Part model, mm, in its own coordinate system. Face numbers are marked on the shaded views. A direction names the side the tool comes from. Coordinates: 2 decimals unless noted, no trailing zeros. Write each loop counter-clockwise with the first axis right and the second up, starting at its lowest first coordinate (ties: lowest second). Pieces come first, ordered by that corner, then holes. Notation, with made-up numbers: M -33,-22 L 14,-22 A21 ccw 14,-13 Z; hole C 25,-22 d6. An arc over 180 degrees is marked long. Use a Markdown table: item, result. Add a question column.
Q1. Slice it at C-C on z = -27. Write the cut outline in (x, y), then the cut area to 3 significant figures.
Q2. Pin check, flat tips, straight feed: pin 1 Ø5 at (y, z) = (-17.5, -44.5) entering from -X; pin 2 Ø18.5 at (x, z) = (20, -32.5) entering from -Y. Stop position of each tip, or through.
Q3. Slice it at D-D on y = -11. Write the cut outline in (x, z), then the cut area to 3 significant figures.
Q4. Slice it at A-A on z = -44.5. Write the cut outline in (x, y), then the cut area to 3 significant figures.
Q5. Wall check: L1, parallel to Z at x = 38.7, y = -24.5; L2, parallel to Z at x = 38, y = -13.5; L3, parallel to Y at x = 29.5, z = -41.5. Give the ranges that are in metal, low to high. Write a range as from..to.
Q6. Slice it at B-B on y = -21. Write the cut outline in (x, z), then the cut area to 3 significant figures.
Q7. Tool access for the marked faces 1 and 2: list every direction of +Z, -Z, +X, -X, +Y, -Y with a clear straight run to the whole face (end or side of a thin tool).
from build123d import *

# Parameters (mm, degrees)
SKETCH_1_W          = 40
SKETCH_1_H          = 40
EXTRUDE_1_DEPTH     = 80
SHELL_1_T           = -3
SKETCH_2_R          = 1.5
CUT_EXTRUDE_1_DEPTH = 98.979589711
SKETCH_3_R          = 2
CUT_EXTRUDE_2_DEPTH = 80


with BuildPart() as part:
    # 草图1 → 凸台-拉伸1 (new body)
    with BuildSketch(Plane.XY):
        with Locations((20, -20)):
            Rectangle(SKETCH_1_W, SKETCH_1_H)
    extrude(amount=-EXTRUDE_1_DEPTH)

    # 抽壳1
    shell_1_openings = [part.faces().sort_by_distance(p)[0] for p in [
        (20, -20, -80),
        (20, -20, 0),
        (20, -40, -40),
        (0, -20, -40),
    ]]
    offset(amount=SHELL_1_T, openings=shell_1_openings, kind=Kind.INTERSECTION)

    # 草图2 → 切除-拉伸1 (cut, through all)
    with BuildSketch(Plane(origin=(40, 0, 0), x_dir=(0, 0, -1), z_dir=(1, 0, 0))):
        with Locations(Location((44.5, -17.5, 0), (0, 0, 90))):
            Circle(SKETCH_2_R)
        with Locations(Location((27, -21, 0), (0, 0, 90))):
            Circle(SKETCH_2_R)
        with Locations(Location((34, -28, 0), (0, 0, 90))):
            Circle(SKETCH_2_R)
        with Locations(Location((27, -35, 0), (0, 0, 90))):
            Circle(SKETCH_2_R)
        with Locations(Location((20, -28, 0), (0, 0, 90))):
            Circle(SKETCH_2_R)
        with Locations(Location((73.5, -13.5, 0), (0, 0, 90))):
            Circle(SKETCH_2_R)
        with Locations(Location((16.5, -10.5, 0), (0, 0, 90))):
            Circle(SKETCH_2_R)
        with Locations(Location((23.5, -17.5, 0), (0, 0, 90))):
            Circle(SKETCH_2_R)
        with Locations(Location((9.5, -17.5, 0), (0, 0, 90))):
            Circle(SKETCH_2_R)
        with Locations(Location((16.5, -24.5, 0), (0, 0, 90))):
            Circle(SKETCH_2_R)
        with Locations(Location((37.5, -24.5, 0), (0, 0, 90))):
            Circle(SKETCH_2_R)
        with Locations(Location((30.5, -17.5, 0), (0, 0, 90))):
            Circle(SKETCH_2_R)
        with Locations(Location((37.5, -10.5, 0), (0, 0, 90))):
            Circle(SKETCH_2_R)
    extrude(amount=-CUT_EXTRUDE_1_DEPTH, mode=Mode.SUBTRACT)

    # 草图3 → 切除-拉伸2 (cut)
    with BuildSketch(Plane(origin=(0, 0, 0), x_dir=(1, 0, 0), z_dir=(0, 1, 0))):
        with Locations(Location((33, 67.5, 0), (0, 0, 270))):
            Circle(SKETCH_3_R)
    extrude(amount=-CUT_EXTRUDE_2_DEPTH, mode=Mode.SUBTRACT)


solid = part.part
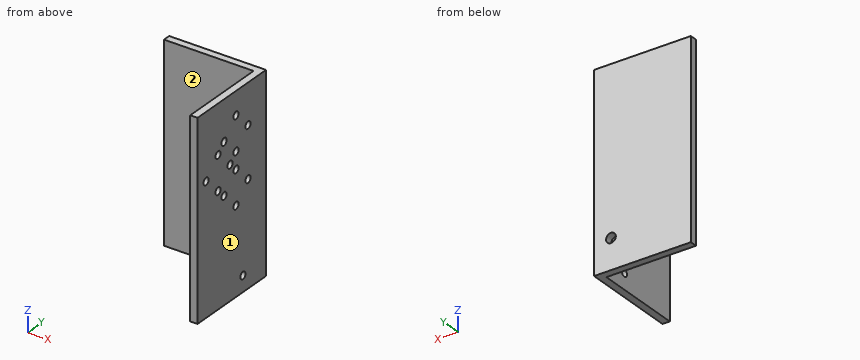
Recorded:
| question | item | result |
|---|---|---|
| 1 | outline | M 0,-3 L 37,-3 L 37,-19.5 L 40,-19.5 L 40,0 L 0,0 Z; M 37,-40 L 40,-40 L 40,-36.5 L 37,-36.5 Z; M 37,-33.5 L 40,-33.5 L 40,-22.5 L 37,-22.5 Z |
| 1 | area | 213 mm² |
| 2 | pin 1 | x = 37 |
| 2 | pin 2 | y = -3 |
| 3 | outline | M 37,-80 L 40,-80 L 40,-38.91 L 37,-38.91 Z; M 37,-36.09 L 40,-36.09 L 40,-17.91 L 37,-17.91 Z; M 37,-15.09 L 40,-15.09 L 40,0 L 37,0 Z |
| 3 | area | 223 mm² |
| 4 | outline | M 0,-3 L 37,-3 L 37,-16 L 40,-16 L 40,0 L 0,0 Z; M 37,-40 L 40,-40 L 40,-19 L 37,-19 Z |
| 4 | area | 222 mm² |
| 5 | L1 | -80..-39, -36..-18, -15..0 |
| 5 | L2 | -80..-75, -72..0 |
| 5 | L3 | -3..0 |
| 6 | outline | M 37,-80 L 40,-80 L 40,-28.5 L 37,-28.5 Z; M 37,-25.5 L 40,-25.5 L 40,0 L 37,0 Z |
| 6 | area | 231 mm² |
| 7 | face 1 | +Z, -Z, +X, +Y, -Y |
| 7 | face 2 | +Z, -Z, -X, -Y |
